from build123d import *

# Parameters (mm, degrees)
BOSS_EXTRUDE2_DEPTH = 8
SKETCH5_R           = 9
CUT_EXTRUDE2_DEPTH  = 8
BOSS_EXTRUDE3_DEPTH = 32
CUT_EXTRUDE3_DEPTH  = 12
SKETCH8_W           = 40
SKETCH8_H           = 10
BOSS_EXTRUDE4_DEPTH = 32
SKETCH10_R          = 15
BOSS_EXTRUDE5_DEPTH = 20
CUT_EXTRUDE4_DEPTH  = 10
CUT_EXTRUDE5_DEPTH  = 10
SKETCH14_R          = 10
CUT_EXTRUDE6_DEPTH  = 20


with BuildPart() as part:
    # Sketch1 → Boss-Extrude2 (new body)
    with BuildSketch(Plane.XY):
        with BuildLine():
            Line((0, 0), (56, 0))
            ThreePointArc((56, 0), (74, 18), (56, 36))
            Line((56, 36), (0, 36))
            ThreePointArc((0, 36), (-18, 18), (0, 0))
        make_face()
    extrude(amount=BOSS_EXTRUDE2_DEPTH)

    # Sketch5 → Cut-Extrude2 (cut)
    with BuildSketch(Plane(origin=(0, 0, 0), x_dir=(-1, 0, 0), z_dir=(0, 0, -1))):
        with Locations((0, 18)):
            Circle(SKETCH5_R)
        with Locations((-56, 18)):
            Circle(SKETCH5_R)
    extrude(amount=-CUT_EXTRUDE2_DEPTH, mode=Mode.SUBTRACT)

    # Sketch6 → Boss-Extrude3 (add)
    with BuildSketch(Plane.XY.offset(8)):
        Polygon((8, 36), (48, 36), (48, 26), (34, 26), (34, 0), (22, 0), (22, 26), (8, 26), align=None)
    extrude(amount=BOSS_EXTRUDE3_DEPTH)

    # Sketch7 → Cut-Extrude3 (cut)
    with BuildSketch(Plane(origin=(34, 0, 0), x_dir=(0, 0, -1), z_dir=(1, 0, 0))):
        Polygon((-40, 26), (-8, 0), (-40, 0), align=None)
    extrude(amount=-CUT_EXTRUDE3_DEPTH, mode=Mode.SUBTRACT)

    # Sketch8 → Boss-Extrude4 (add)
    with BuildSketch(Plane(origin=(0, 36, 0), x_dir=(1, 0, 0), z_dir=(0, 1, 0))):
        with Locations((28, -35)):
            Rectangle(SKETCH8_W, SKETCH8_H)
    extrude(amount=BOSS_EXTRUDE4_DEPTH)

    # Sketch10 → Boss-Extrude5 (add)
    with BuildSketch(Plane(origin=(0, 0, 30), x_dir=(-1, 0, 0), z_dir=(0, 0, -1))):
        with Locations((-28, 68)):
            Circle(SKETCH10_R)
    extrude(amount=-BOSS_EXTRUDE5_DEPTH)

    # Sketch11 → Cut-Extrude4 (cut)
    with BuildSketch(Plane.XY.offset(40)):
        Polygon((43, 68), (48, 36), (48, 68), align=None)
    extrude(amount=-CUT_EXTRUDE4_DEPTH, mode=Mode.SUBTRACT)

    # Sketch13 → Cut-Extrude5 (cut)
    with BuildSketch(Plane.XY.offset(40)):
        Polygon((13, 68), (8, 36), (8, 68), align=None)
    extrude(amount=-CUT_EXTRUDE5_DEPTH, mode=Mode.SUBTRACT)

    # Sketch14 → Cut-Extrude6 (cut)
    with BuildSketch(Plane.XY.offset(50)):
        with Locations((28, 68)):
            Circle(SKETCH14_R)
    extrude(amount=-CUT_EXTRUDE6_DEPTH, mode=Mode.SUBTRACT)


solid = part.part
Read the model definition and answer for the solid it produces. Units are mm, in the model's axes. A direction names the side the tool comes from. Round coordinates to 2 decimals unless told otherwise and drop trailing zeros. Write each loop counter-clockwise with the first axis right and the second up, starting at its lowest first coordinate (ties: lowest second). Pieces come first, ordered by that corner, then holes.
1. The part is cut by section A-A, the plane x = 28. Determine the outline of the cut face in (y, z), then the cut area to 3 significant figures.
2. The part is cut by section D-D, the plane z = 15. Determine the outline of the cut face in (x, y), then the cut area to 3 significant figures.
3. The part is cut by section C-C, the plane z = 38. Determine the outline of the cut face in (x, y) (3 decimals).
4. The part is cut by section B-B, the plane y = 15. Determine the outline of the cut face in (x, z), then the cut area to 3 significant figures.
5. Given pin 1 Ø4 at (x, z) = (43.5, 30.5) entering from -Y; pin 2 Ø1.5 at (y, z) = (61.5, 43) entering from -X; pin 3 Ø2 at (y, z) = (31.5, 22) entering from -X; pin 4 Ø12 at (y, z) = (58, 21) entering from +X, each flat-ended and moving along its own axis, determine where each tip first touches the part or whether it passes through.
6. Which of the six approach directions +Z, -Z, +X, -X, +Y, -Y give full straight-line access (tool end or side, diameter ignored) to faces 4 (the face through (48, 31, 24)), 5 (the face through (8, 31, 24)), 6 (the face through (41, 26, 24)), 7 (the face through (29.953, 82.872, 42.082))?
7. Determine the mould class of faces 1 (the face through (33.38, 76.43, 40.14)), 2 (the face through (74, 18, 4)), 3 (the face through (28, 42, 40)) for opening direction Y: pulls with the +Y half, pulls with the -Y half, needs draft (parallel to the pull), parting line crosses it, or undercut.
8. Straight lines are drawn through the part: L1, parallel to Y at x = 56, z = 6.5; L2, parallel to X at y = 21.5, z = 20; L3, parallel to Y at x = 28, z = 41. For each, find the intervals that lie inside material, in ascending order.
Values:
1. outline: (0, 0) - (36, 0) - (36, 30) - (58, 30) - (58, 50) - (53, 50) - (53, 40) - (26, 40) - (0, 8) - close; (78, 30) - (83, 30) - (83, 50) - (78, 50) - close
1. area: 1,390 mm2
2. outline: (8, 26) - (22, 26) - (22, 5.69) - (34, 5.69) - (34, 26) - (48, 26) - (48, 36) - (8, 36) - close
2. area: 644 mm2
3. outline: (8, 26) - (22, 26) - (22, 24.375) - (34, 24.375) - (34, 26) - (48, 26) - (48, 36) - (43, 68) arc R15 ccw to (13, 68) - (8, 36) - close; hole circle Ø20 at (28, 68)
4. outline: (-17.75, 0) - (-8.49, 0) - (-8.49, 8) - (-17.75, 8) - close; (8.49, 0) - (47.51, 0) - (47.51, 8) - (34, 8) - (34, 26.46) - (22, 26.46) - (22, 8) - (8.49, 8) - close; (64.49, 0) - (73.75, 0) - (73.75, 8) - (64.49, 8) - close
4. area: 682 mm2
5. pin 1: stops at y = 26
5. pin 2: stops at x = 14.15
5. pin 3: stops at x = 8
5. pin 4: passes through
6. face 4: +Z, +X, +Y, -Y
6. face 5: +Z, -X, +Y, -Y
6. face 6: +Z, +X, -Y
6. face 7: +Z
7. face 1: undercut
7. face 2: parting line crosses it
7. face 3: needs draft
8. L1: y = 0 to 9, 27 to 36
8. L2: x = 22 to 34
8. L3: y = 53 to 58, 78 to 83
